from build123d import *

# Parameters (mm, degrees)
F0_R     = 12.5
F0_R_2   = 10
F0_R_3   = 6
F0_R_4   = 5
F0_R_5   = 2.25
F1_DEPTH = 3
F2_DEPTH = 4
F3_DEPTH = 32


with BuildPart() as f1:
    # F0 (on Front) → F1 (new body)
    with BuildSketch(Plane.XZ):
        Circle(F0_R)
        Circle(F0_R_2, mode=Mode.SUBTRACT)
        Circle(F0_R_2)
        Circle(F0_R_3, mode=Mode.SUBTRACT)
        Circle(F0_R_3)
        Circle(F0_R_4, mode=Mode.SUBTRACT)
        Circle(F0_R_4)
        Circle(F0_R_5, mode=Mode.SUBTRACT)
    extrude(amount=F1_DEPTH)

    # F0 (on Front) → F2 (join)
    with BuildSketch(Plane.XZ):
        Circle(F0_R_4)
        Circle(F0_R_5, mode=Mode.SUBTRACT)
    extrude(amount=F2_DEPTH)

    # F0 (on Front) → F3 (join)
    with BuildSketch(Plane.XZ):
        Circle(F0_R_2)
        Circle(F0_R_3, mode=Mode.SUBTRACT)
    extrude(amount=F3_DEPTH)


solid = f1.part
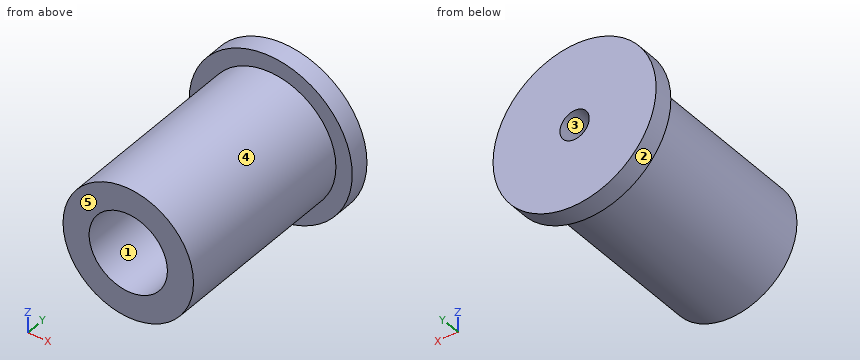
Geometry: final body of the model. Coordinates: model frame, mm. Face numbers are marked on the shaded views. A direction names the side the tool comes from. Coordinates: 2 decimals unless noted, no trailing zeros. Loops run counter-clockwise (first coordinate to the right, second up) from the corner with the lowest first, then second, coordinate; pieces in that order, holes last. Notation, with made-up numbers: (17, 9.25) - (57, 9.25) arc R27 ccw to (57, 44.25) - close; hole circle Ø7 at (-4.75, 23.25). An arc over 180 degrees is marked (long way). Put each result on its own line as item: value. Start each with the question number.
Q1. Line query: line 1 (Z direction, x = 0, y = -1.1); line 2 (Z direction, x = 0, y = -19.25). Output: solid intervals per line, ascending.
Q2. Pin query (flat end, axial travel): pin 1 Ø1 at (x, z) = (-8, 9.5) entering from -Y; pin 2 Ø12 at (x, y) = (-7.5, -3.5) entering from +Z; pin 3 Ø5 at (y, z) = (-16.5, 3.5) entering from +X. Return the tip coordinate at first contact, or that it passes through.
Q3. Set-up query: the marked faces 1 and 2. Return all of +Z, -Z, +X, -X, +Y, -Y with unobstructed straight access to the full face (end or side cutting, diameter ignored); none if empty.
Q4. Cut plane C-C, the plane y = -3.5. Return loops of the section in (x, z).
Q5. Cut plane B-B, the plane x = 0. Return loops of the section in (y, z), and give its area (3 significant figures).
Q6. Cut plane A-A, the plane z = 0. Return loops of the section in (x, y), and give its area (3 significant figures).
Q7. Cut plane D-D, the plane y = -26.5. Return loops of the section in (x, z).
Q8. Pull-direction query (Z, two-part tool) for the marked faces 3, 4 and 5; classes: released by +Z, released by -Z, zero draft, split by the parting line, or undercut.
Filled sheet:
1. line 1: -12.5 to -2.25, 2.25 to 12.5
1. line 2: -10 to -6, 6 to 10
2. pin 1: y = -3
2. pin 2: z = 12.41
2. pin 3: x = 9.95
3. face 1: -Y
3. face 2: +Y, -Y
4. outline: circle Ø20 at (0, 0); circle Ø10 at (0, 0); hole circle Ø12 at (0, 0); hole circle Ø4.5 at (0, 0)
5. outline: (-32, -10) - (-3, -10) - (-3, -12.5) - (0, -12.5) - (0, -2.25) - (-4, -2.25) - (-4, -5) - (-3, -5) - (-3, -6) - (-32, -6) - close; (-32, 6) - (-3, 6) - (-3, 5) - (-4, 5) - (-4, 2.25) - (0, 2.25) - (0, 12.5) - (-3, 12.5) - (-3, 10) - (-32, 10) - close
5. area: 299 mm²
6. outline: (-12.5, -3) - (-10, -3) - (-10, -32) - (-6, -32) - (-6, -3) - (-5, -3) - (-5, -4) - (-2.25, -4) - (-2.25, 0) - (-12.5, 0) - close; (2.25, -4) - (5, -4) - (5, -3) - (6, -3) - (6, -32) - (10, -32) - (10, -3) - (12.5, -3) - (12.5, 0) - (2.25, 0) - close
6. area: 299 mm²
7. outline: circle Ø20 at (0, 0); hole circle Ø12 at (0, 0)
8. face 3: undercut
8. face 4: split by the parting line
8. face 5: zero draft
